from build123d import *

# Parameters (mm, degrees)
CROQUIS1_W                   = 50
CROQUIS1_H                   = 60
SALIENTE_EXTRUIR1_DEPTH      = 50
VACIADO1_T                   = -3
CROQUIS2_W                   = 12.2
CROQUIS2_H                   = 4.8
CROQUIS2_R                   = 0.9
SALIENTE_EXTRUIR2_DEPTH      = 18.3
CORTAR_EXTRUIR1_REACH        = 71.148
CORTAR_EXTRUIR2_START        = 18.3
CROQUIS2_3_R                 = 0.9
CORTAR_EXTRUIR2_DEPTH        = 8
CORTAR_EXTRUIR3_DEPTH        = 64.442887702
CORTAR_EXTRUIR3_DEPTH_BACK   = 2.4
CROQUIS5_W                   = 47
CROQUIS5_H                   = 57
REDONDEO1_R                  = 0.5
CHAFL_N1_SIZE                = 0.5
SALIENTE_EXTRUIR3_DEPTH      = 3
NGULO_DE_SALIDA5_ANGLE       = 1
REDONDEO3_R                  = 5
TALADROAVANZADO1_START       = 1.55
TALADROAVANZADO1_OUTLINE_R   = 4
TALADROAVANZADO1_DEPTH       = 1.45
TALADROAVANZADO1_2_OUTLINE_R = 1.7
TALADROAVANZADO1_2_DEPTH     = 1.55
NERVIO4_START                = -0.9
NERVIO4_DEPTH                = 1.8
NERVIO5_REACH                = 86.436
CROQUIS16_WALL_W             = 7.071067812
CROQUIS16_WALL_H             = 1.8
CORTAR_EXTRUIR8_DEPTH        = 68.975657408
CORTAR_EXTRUIR8_DEPTH_BACK   = 13
NERVIO9_START                = -3
NERVIO9_OUTLINE_W            = 31.268599093
NERVIO9_OUTLINE_H            = 39.871788568
NERVIO9_DEPTH                = 3
REDONDEO4_R                  = 2
REDONDEO5_R                  = 2
CORTAR_EXTRUIR9_REACH        = 102.177


# Read off the part's stored shape, not the designer's step: TaladroAvanzado1, Nervio4, Nervio9
with BuildPart() as part:
    # Croquis1 → Saliente-Extruir1 (new body)
    with BuildSketch(Plane(origin=(0, 0, 0), x_dir=(1, 0, 0), z_dir=(0, 1, 0))):
        Rectangle(CROQUIS1_W, CROQUIS1_H)
    extrude(amount=SALIENTE_EXTRUIR1_DEPTH)

    # Vaciado1
    vaciado1_openings = [part.faces().sort_by_distance(p)[0] for p in [
        (0, 50, 0),
    ]]
    offset(amount=VACIADO1_T, openings=vaciado1_openings, kind=Kind.INTERSECTION)

    # Croquis2 → Saliente-Extruir2 (add)
    # profile 1 of 2: a face of its own
    with BuildSketch(Plane(origin=(0, 3, 0), x_dir=(1, 0, 0), z_dir=(0, 1, 0))):
        with Locations((0, 8.3)):
            Rectangle(CROQUIS2_W, CROQUIS2_H)
    # profile 2 of 2: a face of its own
    with BuildSketch(Plane(origin=(0, 3, 0), x_dir=(1, 0, 0), z_dir=(0, 1, 0))):
        with Locations((0, -19.4)):
            Rectangle(CROQUIS2_W, CROQUIS2_H)
        with Locations(Location((0, -19.55, 0), (0, 0, 270))):
            Circle(CROQUIS2_R, mode=Mode.SUBTRACT)
    extrude(amount=SALIENTE_EXTRUIR2_DEPTH)

    # Croquis4 → Cortar-Extruir1 (cut, up to next)
    with BuildSketch(Plane(origin=(0, 0, -10.7), x_dir=(-1, 0, 0), z_dir=(0, 0, -1)), mode=Mode.PRIVATE) as cortar_extruir1_sk1:
        with BuildLine():
            Line((-3.7, 3), (3.7, 3))
            Line((3.7, 3), (3.7, 7.5))
            ThreePointArc((3.7, 7.5), (0, 11.2), (-3.7, 7.5))
            Line((-3.7, 7.5), (-3.7, 3))
        make_face()
    cortar_extruir1_tool1 = extrude(cortar_extruir1_sk1.sketch, amount=-CORTAR_EXTRUIR1_REACH, mode=Mode.PRIVATE) & part.part
    add(cortar_extruir1_tool1.solids().sort_by_distance((0, 6.74903, -10.7))[0], mode=Mode.SUBTRACT)

    # Croquis2<3> → Cortar-Extruir2 (cut)
    with BuildSketch(Plane(origin=(0, 3, 0), x_dir=(1, 0, 0), z_dir=(0, 1, 0)).offset(CORTAR_EXTRUIR2_START)):
        with Locations(Location((0, 8.45, 0), (0, 0, 270))):
            Circle(CROQUIS2_3_R)
    extrude(amount=-CORTAR_EXTRUIR2_DEPTH, mode=Mode.SUBTRACT)

    # Croquis5 → Cortar-Extruir3 (cut, two sides: drawn at the far end of the back side and taken through both)
    with BuildSketch(Plane(origin=(0, 50, 0), x_dir=(1, 0, 0), z_dir=(0, 1, 0)).offset(-CORTAR_EXTRUIR3_DEPTH_BACK)):
        Rectangle(CROQUIS5_W, CROQUIS5_H)
    extrude(amount=CORTAR_EXTRUIR3_DEPTH + CORTAR_EXTRUIR3_DEPTH_BACK, mode=Mode.SUBTRACT)

    # Redondeo1
    redondeo1_edges = [part.edges().sort_by_distance(p)[0] for p in [
        (0, 47.6, 28.5),
        (23.5, 47.6, 0),
        (0, 47.6, -28.5),
        (-23.5, 47.6, 0),
    ]]
    fillet(redondeo1_edges, radius=REDONDEO1_R)

    # Chaflán1
    chafl_n1_edges = [part.edges().sort_by_distance(p)[0] for p in [
        (0, 50, 28.5),
        (23.5, 50, 0),
        (0, 50, -28.5),
        (-23.5, 50, 0),
    ]]
    chamfer(chafl_n1_edges, length=CHAFL_N1_SIZE)

    # Croquis11 → Saliente-Extruir3 (add)
    with BuildSketch(Plane.XZ):
        with BuildLine():
            Line((-25, 6), (-35, 6))
            ThreePointArc((-35, 6), (-41, 0), (-35, -6))
            Line((-35, -6), (-25, -6))
            Line((-25, -6), (-25, 6))
        make_face()
        with BuildLine():
            Line((25, 6), (35, 6))
            ThreePointArc((35, 6), (41, 0), (35, -6))
            Line((35, -6), (25, -6))
            Line((25, -6), (25, 6))
        make_face()
        with BuildLine():
            Line((6, -30), (-6, -30))
            Line((-6, -30), (-6, -40))
            ThreePointArc((-6, -40), (0, -46), (6, -40))
            Line((6, -40), (6, -30))
        make_face()
        with BuildLine():
            Line((-6, 30), (6, 30))
            Line((6, 30), (6, 40))
            ThreePointArc((6, 40), (0, 46), (-6, 40))
            Line((-6, 40), (-6, 30))
        make_face()
    extrude(amount=-SALIENTE_EXTRUIR3_DEPTH)

    # Ángulo de salida5
    ngulo_de_salida5_faces = [part.faces().sort_by_distance(p)[0] for p in [
        (25, 25.285425101, 0),
        (0, 25.343344156, 30),
        (-25, 25.285425101, 0),
        (0, 25.343344156, -30),
    ]]
    draft(ngulo_de_salida5_faces, Plane.ZX.offset(50), NGULO_DE_SALIDA5_ANGLE)

    # Redondeo3
    redondeo3_edges = [part.edges().sort_by_distance(p)[0] for p in [
        (-25.820388052, 3, 0),
        (25.820388052, 3, 0),
        (0, 3, -30.820388052),
        (0, 3, 30.820388052),
    ]]
    fillet(redondeo3_edges, radius=REDONDEO3_R)

    # TaladroAvanzado1 outline → TaladroAvanzado1 (cut)
    with BuildSketch(Plane(origin=(0, 0, 0), x_dir=(1, 0, 0), z_dir=(0, 1, 0)).offset(TALADROAVANZADO1_START)):
        with Locations((0, -40)):
            Circle(TALADROAVANZADO1_OUTLINE_R)
        with Locations((0, 40)):
            Circle(TALADROAVANZADO1_OUTLINE_R)
        with Locations((-35, 0)):
            Circle(TALADROAVANZADO1_OUTLINE_R)
        with Locations((35, 0)):
            Circle(TALADROAVANZADO1_OUTLINE_R)
    extrude(amount=TALADROAVANZADO1_DEPTH, mode=Mode.SUBTRACT)

    # TaladroAvanzado1 2 outline → TaladroAvanzado1 2 (cut)
    with BuildSketch(Plane(origin=(0, 0, 0), x_dir=(1, 0, 0), z_dir=(0, 1, 0))):
        with Locations((0, -40)):
            Circle(TALADROAVANZADO1_2_OUTLINE_R)
        with Locations((0, 40)):
            Circle(TALADROAVANZADO1_2_OUTLINE_R)
        with Locations((-35, 0)):
            Circle(TALADROAVANZADO1_2_OUTLINE_R)
        with Locations((35, 0)):
            Circle(TALADROAVANZADO1_2_OUTLINE_R)
    extrude(amount=TALADROAVANZADO1_2_DEPTH, mode=Mode.SUBTRACT)

    # Nervio4 outline → Nervio4 (add)
    with BuildSketch(Plane(origin=(0, 0, 19.4), x_dir=(-1, 0, 0), z_dir=(0, 0, -1)).offset(NERVIO4_START)):
        Polygon((11.1, 3), (6.1, 8), (6.1, 3), align=None)
    nervio4 = extrude(amount=NERVIO4_DEPTH)

    # Simetría1: Nervio4 across plane
    add(nervio4.mirror(Plane(origin=(0, 0, 0), x_dir=(0, 0, 1), z_dir=(1, 0, 0))))

    # Croquis16 wall → Nervio5 (add, up to next)
    with BuildSketch(Plane(origin=(-8.6, 5.5, -8.3), x_dir=(-0.707106781187, -0.707106781187, 0), z_dir=(-0.707106781187, 0.707106781187, 0)), mode=Mode.PRIVATE) as nervio5_sk1:
        Rectangle(CROQUIS16_WALL_W, CROQUIS16_WALL_H)
    nervio5_tool1 = extrude(nervio5_sk1.sketch, amount=-NERVIO5_REACH, mode=Mode.PRIVATE) - part.part
    nervio5 = nervio5_tool1.solids().sort_by_distance((-8.6, 5.5, -8.3))[0]
    add(nervio5)

    # Simetría2: Nervio5 across plane
    add(nervio5.mirror(Plane(origin=(0, 0, 0), x_dir=(0, 0, 1), z_dir=(1, 0, 0))))

    # Croquis17 → Cortar-Extruir8 (cut, two sides: drawn at the far end of the back side and taken through both)
    with BuildSketch(Plane(origin=(0, 21.3, 0), x_dir=(1, 0, 0), z_dir=(0, 1, 0)).offset(-CORTAR_EXTRUIR8_DEPTH_BACK)):
        with BuildLine():
            ThreePointArc((3.512549094, 5.9), (0, 6.52196544), (-3.512549094, 5.9))
            Line((-3.512549094, 5.9), (3.512549094, 5.9))
        make_face()
    extrude(amount=CORTAR_EXTRUIR8_DEPTH + CORTAR_EXTRUIR8_DEPTH_BACK, mode=Mode.SUBTRACT)

    # Nervio9 outline → Nervio9 (add)
    with BuildSketch(Plane(origin=(0, 6, 0), x_dir=(1, 0, 0), z_dir=(0, 1, 0)).offset(NERVIO9_START)):
        Polygon((-22, -12.74799793), (-18.968599093, -12.74799793), (-18.968599093, -23.546859472), (-22, -23.546859472), (-22, -25.346859472), (14.1, -25.346859472), (14.1, -27), (15.9, -27), (15.9, -25.346859472), (22, -25.346859472), (22, -23.546859472), (15.9, -23.546859472), (15.9, -13.648622413), (22, -13.648622413), (22, -11.848622413), (15.9, -11.848622413), (15.9, -7.199306775), (22, -7.199306775), (22, -5.399306775), (15.9, -5.399306775), (15.9, -0.9), (22, -0.9), (22, 0.9), (15.9, 0.9), (15.9, 7.38606859), (22, 7.38606859), (22, 9.18606859), (15.9, 9.18606859), (15.9, 16.324929096), (22, 16.324929096), (22, 18.124929096), (15.9, 18.124929096), (15.9, 27), (14.1, 27), (14.1, 18.124929096), (5.7899715, 18.124929096), (5.7899715, 27), (3.9899715, 27), (3.9899715, 18.124929096), (-7.13941805, 18.124929096), (-7.13941805, 27), (-8.93941805, 27), (-8.93941805, 18.124929096), (-17.168599093, 18.124929096), (-17.168599093, 27), (-18.968599093, 27), (-18.968599093, 9.18606859), (-22, 9.18606859), (-22, 7.38606859), (-18.968599093, 7.38606859), (-18.968599093, 0.9), (-22, 0.9), (-22, -0.9), (-18.968599093, -0.9), (-18.968599093, -5.399306775), (-22, -5.399306775), (-22, -7.199306775), (-18.968599093, -7.199306775), (-18.968599093, -10.94799793), (-22, -10.94799793), align=None)
        with Locations((-1.534299546, -3.610965188)):
            Rectangle(NERVIO9_OUTLINE_W, NERVIO9_OUTLINE_H, mode=Mode.SUBTRACT)
    extrude(amount=NERVIO9_DEPTH)

    # Redondeo4
    redondeo4_edges = [part.edges().sort_by_distance(p)[0] for p in [
        (25.436376623, 25, 30.436376623),
        (-25.436376623, 25, 30.436376623),
        (-25.436376623, 25, -30.436376623),
        (25.436376623, 25, -30.436376623),
    ]]
    fillet(redondeo4_edges, radius=REDONDEO4_R)

    # Redondeo5
    redondeo5_edges = [part.edges().sort_by_distance(p)[0] for p in [
        (-22, 25.3, 27),
        (-22, 25.3, -27),
        (22, 25.3, -27),
        (22, 25.3, 27),
    ]]
    fillet(redondeo5_edges, radius=REDONDEO5_R)

    # Cortar-Extruir9: up to this plane
    cortar_extruir9_end = Plane(origin=(-25, 50, -27), z_dir=(0, 0, 1))
    # Croquis21 → Cortar-Extruir9 (cut, up to the surface)
    with BuildSketch(Plane(origin=(0, 0.538721775, -30.863349823), x_dir=(-1, 0, 0), z_dir=(0, 0.01745240643728355, -0.9998476951563913)), mode=Mode.PRIVATE) as cortar_extruir9_sk1:
        with BuildLine():
            Line((12, 5.461196163), (20, 5.461196163))
            Line((20, 5.461196163), (20, 11.461196163))
            ThreePointArc((20, 11.461196163), (16, 15.461196163), (12, 11.461196163))
            Line((12, 11.461196163), (12, 5.461196163))
        make_face()
    cortar_extruir9_tool1 = split(extrude(cortar_extruir9_sk1.sketch, amount=-CORTAR_EXTRUIR9_REACH, mode=Mode.PRIVATE), bisect_by=cortar_extruir9_end, keep=Keep.BOTH, mode=Mode.PRIVATE)
    add(cortar_extruir9_tool1.solids().sort_by_distance((-16, 10.612775, -30.687507))[0], mode=Mode.SUBTRACT)


solid = part.part
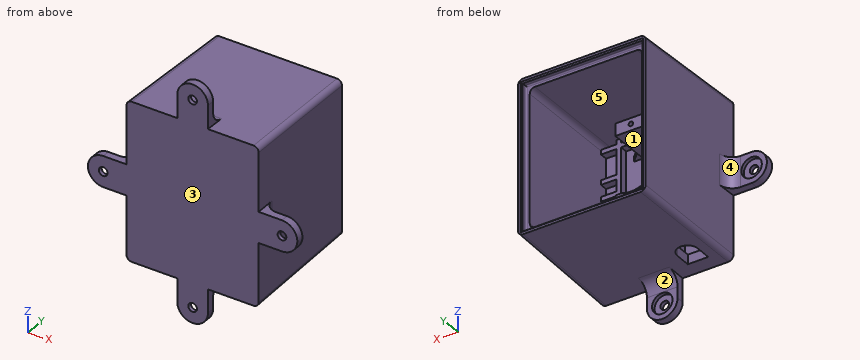
Verification items for the finished model (mm, model axes). Face numbers are marked on the shaded views. A direction names the side the tool comes from. Round coordinates to 2 decimals unless told otherwise and drop trailing zeros.
(1) Access from +Z, -Z, +X, -X, +Y, -Y to the whole of each face (thin tool, end or side, straight path). Record for the marked faces 4 and 5.
Returned:
face 4: +Z, -Z, -X, +Y
face 5: +Y
(2) Mould release check, pull along Z, two halves, no side actions. Record for the marked faces 1, 2 and 3: pulls with the +Z half, pulls with the -Z half, needs draft (parallel to the pull), parting line crosses it, or undercut.
Returned:
face 1: undercut
face 2: pulls with the -Z half
face 3: needs draft
(3) Depth check by flat-ended pin: pin 1 Ø1.1 at (x, y) = (-19.5, 5) entering from +Z; pin 2 Ø0.7 at (x, y) = (4.5, 48.5) entering from -Z; pin 3 Ø8 at (x, z) = (-2.5, 41.5) entering from +Y. Enter the tip coordinate at first touch or a pass-through.
Returned:
pin 1: stops at z = 30.8
pin 2: stops at z = -30.03
pin 3: stops at y = 3
(4) Material ranges on line 1 (Z direction, x = 0, y = 1); line 2 (X direction, y = 1.2, z = 0); line 3 (Z direction, x = 35, y = 1.05), recorded low to high.
Returned:
line 1: z = -46 to -41.7, -38.3 to 38.3, 41.7 to 46
line 2: x = -41 to -36.7, -33.3 to 33.3, 36.7 to 41
line 3: z = -6 to -1.7, 1.7 to 6
